Design review of the part built by this model. Coordinates are the model's own, in mm. Give positions to 0.01 mm unless a question says otherwise; leave off trailing zeros. Write each loop counter-clockwise with the first axis right and the second up, starting at its lowest first coordinate (ties: lowest second). Pieces come first, ordered by that corner, then holes. Notation, with made-up numbers: M -23.75,50.5 L 18.25,50.5 A37 ccw 18.25,87.5 Z; hole C -0.75,55 d8. An arc over 180 degrees is marked long. Use one line per item in the form item = value. Start each with the question number.
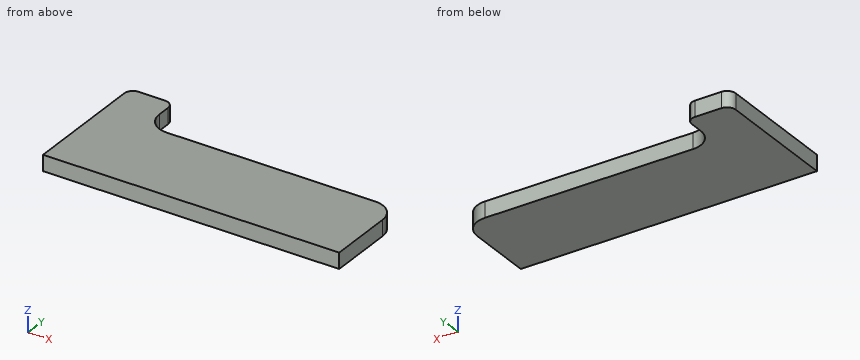
Autodesk Inventor part; units mm, degrees
ref_plane "YZ Plane" through (0, 0, 0) normal (1, 0, 0) x (0, 1, 0)
ref_plane "XZ Plane" through (0, 0, 0) normal (0, 1, 0) x (-1, 0, 0)
ref_plane "XY Plane" through (0, 0, 0) normal (0, 0, 1) x (1, 0, 0)
ref_plane "Work Plane1" through (0, 0, 0) normal (0, 0, 1) x (1, 0, 0)
sketch "Sketch1" plane through (0, 0, 0) normal (0, 0, 1) x (1, 0, 0)
  line L0 (0, 0) -> (675, 0)
  line L1 (675, 0) -> (675, 150)
  line L2 (100, 150) -> (675, 150)
  line L3 (100, 150) -> (100, 850)
  line L4 (0, 850) -> (100, 850)
  line L5 (0, 0) -> (0, 850)
  line L6 (0, 0) -> (100, 0)
  line L7 (80, 300) -> (20, 300)
  line L8 (0, 280) -> (0, 0)
  line L9 (100, 0) -> (675, 0)
  line L10 (675, 0) -> (675, 150)
  line L11 (625, 200) -> (150, 200)
  line L12 (100, 200) -> (100, 0)
  line L13 (100, 0) -> (100, 150)
  line L14 (100, 250) -> (100, 280)
  arc A0 (100, 280) -> (80, 300) centre (80, 280) ccw
  arc A1 (20, 300) -> (0, 280) centre (20, 280) ccw
  arc A2 (675, 150) -> (625, 200) centre (625, 150) ccw
  arc A3 (100, 250) -> (150, 200) centre (150, 250) ccw
  point P0 (100, 300)
  point P1 (0, 300)
  point P2 (675, 200)
  dimension "d0" = 150
  dimension "d1" = 200
  dimension "d2" = 300
  dimension "d3" = 20
  dimension "d4" = 20
  dimension "d5" = 50
extrude "Extrusion1" add sketch "Sketch1" along normal blind 36 contours L5 A1 L7 A0 L3 L12 L0 | L12 L2 L1 L0 | L3 A3 L11 A2 L2
properties part number "bracera"
1. Clearance check with flat-ended pins moving along their axes: pin 1 Ø3 at (x, z) = (449.5, 19) entering from -Y; pin 2 Ø9 at (y, z) = (272, 12) entering from +X; pin 3 Ø10 at (x, z) = (345, 32.5) entering from +Y. State where each tip first meets the part, or that it passes through.
2. We need section B-B (x = 611.5). State the section outline as (y, z) points, and give its area (3 significant figures).
3. We need section C-C (y = 228). State the section outline as (x, z) points.
4. To check wall thickness, follow L1, parallel to Y at x = 411.5, z = 28; L2, parallel to X at y = 270.5, z = 33.5; L3, parallel to X at y = 168, z = 5. State the ranges of each line that lie inside material, in increasing order.
5. We need section A-A (z = 30.5). State the section outline as (x, y) points.
Answer block:
q1.pin_1 = 0
q1.pin_2 = 100
q1.pin_3 = 200
q2.outline = M 0,0 L 200,0 L 200,36 L 0,36 Z
q2.area = 7,200 mm^2
q3.outline = M 0,0 L 105.1,0 L 105.1,36 L 0,36 Z
q4.L1 = 0 to 200
q4.L2 = 0 to 100
q4.L3 = 0 to 671.65
q5.outline = M 0,0 L 675,0 L 675,150 A50 ccw 625,200 L 150,200 A50 cw 100,250 L 100,280 A20 ccw 80,300 L 20,300 A20 ccw 0,280 Z
